from build123d import *

# Parameters (mm, degrees)
F0_W     = 15.14
F0_H     = 18.26
F3_DEPTH = 30.95
F1_W     = 12.5
F1_H     = 5.05
F1_W_2   = 10.5
F1_H_2   = 1.8
F1_R     = 4.635
F4_DEPTH = 12.7
F1_R_2   = 0.425
F1_W_3   = 1.7
F1_H_3   = 2.976594
F2_DEPTH = 12.7


with BuildPart() as f3:
    # F0 (on Top) → F3 (new body)
    with BuildSketch(Plane.XY):
        Rectangle(F0_W, F0_H)
    extrude(amount=F3_DEPTH)

    # F1 (on face) → F4 (cut)
    with BuildSketch(Plane.XZ.offset(9.13)):
        with Locations((0, 26.575)):
            Rectangle(F1_W, F1_H)
        with Locations((0, 27.4)):
            Rectangle(F1_W_2, F1_H_2, mode=Mode.SUBTRACT)
        with Locations((0, 18.075)):
            Rectangle(F1_W, F1_H)
        with Locations((0, 18.9)):
            Rectangle(F1_W_2, F1_H_2, mode=Mode.SUBTRACT)
        with Locations((0, 6.9)):
            Circle(F1_R)
        with BuildLine():
            ThreePointArc((-3.403771, 4.996229), (-3.620699, 8.349324), (-1.15, 10.626594))
            Line((-1.15, 10.626594), (-0.85, 10.626594))
            Line((-0.85, 10.626594), (-0.85, 9.876594))
            Line((-0.85, 9.876594), (0.85, 9.876594))
            Line((0.85, 9.876594), (0.85, 10.626594))
            Line((0.85, 10.626594), (1.15, 10.626594))
            ThreePointArc((1.15, 10.626594), (3.620699, 8.349324), (3.403771, 4.996229))
            Line((3.403771, 4.996229), (1.903771, 4.996229))
            Line((1.903771, 4.996229), (1.903771, 3.496229))
            ThreePointArc((1.903771, 3.496229), (0, 3), (-1.903771, 3.496229))
            Line((-1.903771, 3.496229), (-1.903771, 4.996229))
            Line((-1.903771, 4.996229), (-3.403771, 4.996229))
        make_face(mode=Mode.SUBTRACT)
    extrude(amount=-F4_DEPTH, mode=Mode.SUBTRACT)

    # F1 (on face) → F2 (cut)
    with BuildSketch(Plane.XZ.offset(9.13)):
        with Locations((-2, 8.851594)):
            Circle(F1_R_2)
        with Locations((-2.724793, 6.3)):
            Circle(F1_R_2)
        with Locations((-0.85, 4.246229)):
            Circle(F1_R_2)
        with Locations((2.724793, 6.3)):
            Circle(F1_R_2)
        with Locations((2, 8.851594)):
            Circle(F1_R_2)
        with Locations((0.85, 4.246229)):
            Circle(F1_R_2)
        with Locations((0, 7.788297)):
            Rectangle(F1_W_3, F1_H_3)
    extrude(amount=-F2_DEPTH, mode=Mode.SUBTRACT)


solid = f3.part
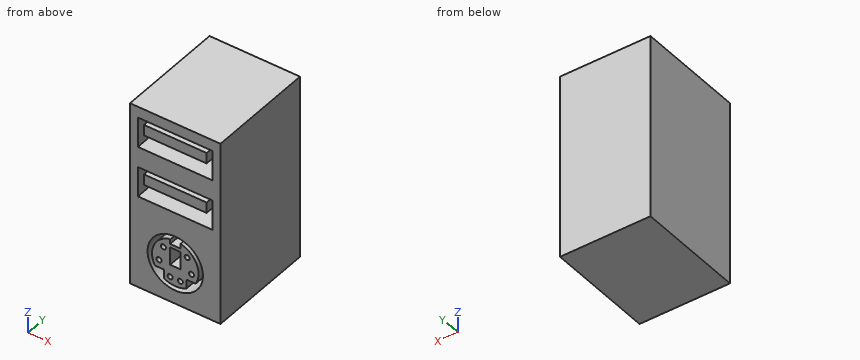
Geometry check sheet. Reference: the model listing, model coordinates, mm. Round coordinates to 2 decimals unless told otherwise and drop trailing zeros. Loops run counter-clockwise (first coordinate to the right, second up) from the corner with the lowest first, then second, coordinate; pieces in that order, holes last.
Item 1: Cross-section at B-B on z = 27.5. Record the boundary of the cut face in (x, y).
Item 2: Cross-section at C-C on y = 1.75. Count the separate pieces of the cut face and the enclosed holes in it, then the cut area to 3 significant figures.
Item 3: Thickness scan on line 1 (X direction, y = 3.5, z = 18.5); line 2 (Z direction, x = 4.75, y = 2.25); line 3 (X direction, y = -7.25, z = 7). Record the ranges inside material, lowest first.
Answer sheet:
1. outline: (-7.57, -9.13) - (-6.25, -9.13) - (-6.25, 3.57) - (-5.25, 3.57) - (-5.25, -9.13) - (5.25, -9.13) - (5.25, 3.57) - (6.25, 3.57) - (6.25, -9.13) - (7.57, -9.13) - (7.57, 9.13) - (-7.57, 9.13) - close
2. separate pieces: 4
2. enclosed holes: 10
2. area: 348 mm2
3. line 1: x = -7.57 to -6.25, -5.25 to 5.25, 6.25 to 7.57
3. line 2: z = 0 to 15.55, 18 to 19.8, 20.6 to 24.05, 26.5 to 28.3, 29.1 to 30.95
3. line 3: x = -7.57 to -4.63, -3.9 to -0.85, 0.85 to 3.9, 4.63 to 7.57
